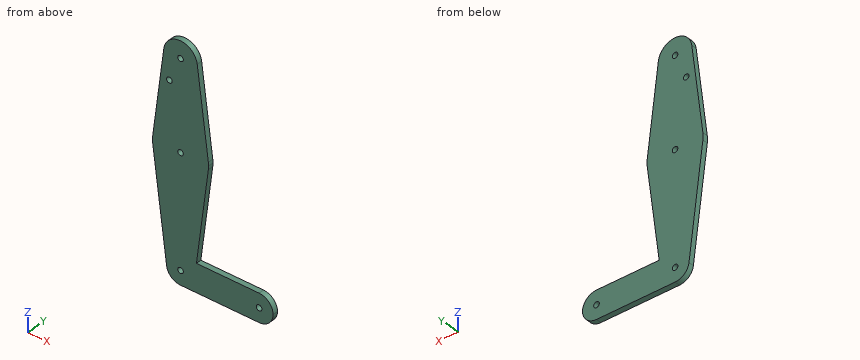
from build123d import *

# Parameters (mm, degrees)
F0_R     = 1.5875
F0_R_2   = 1.6002
F1_DEPTH = 3.048
F4_DEPTH = 3.048


# Not quite as in the source:
# - a feature of the source that left no trace in its solid (it failed there, or was rolled back) is left out


with BuildPart() as f1:
    # F0 (on Front) → F1 (new body)
    with BuildSketch(Plane.XZ):
        with BuildLine():
            ThreePointArc((-9.4502929642, 115.490625), (-0.596483242, 104.7936951058), (9.525, 114.3))
            ThreePointArc((9.525, 114.3), (9.5063048942, 114.896483242), (9.4502929642, 115.490625))
            ThreePointArc((9.4502929642, 115.490625), (0, 123.825), (-9.4502929642, 115.490625))
        make_face()
        with Locations((0, 114.3)):
            Circle(F0_R, mode=Mode.SUBTRACT)
        with BuildLine():
            ThreePointArc((9.4502929642, 115.490625), (9.5063048942, 114.896483242), (9.525, 114.3))
            ThreePointArc((9.525, 114.3), (-0.596483242, 104.7936951058), (-9.4502929642, 115.490625))
            Line((-9.4502929642, 115.490625), (-15.7504882737, 65.484375))
            ThreePointArc((-15.7504882737, 65.484375), (0, 79.375), (15.7504882737, 65.484375))
            Line((15.7504882737, 65.484375), (9.4502929642, 115.490625))
        make_face()
        with Locations((-6.3295518048, 99.7836068273)):
            Circle(F0_R, mode=Mode.SUBTRACT)
        with BuildLine():
            ThreePointArc((15.875, 63.5), (15.8438414904, 64.4941387366), (15.7504882737, 65.484375))
            ThreePointArc((15.7504882737, 65.484375), (0, 79.375), (-15.7504882737, 65.484375))
            ThreePointArc((-15.7504882737, 65.484375), (-15.875, 63.5), (-15.7504882737, 61.515625))
            ThreePointArc((-15.7504882737, 61.515625), (0, 47.625), (15.7504882737, 61.515625))
            ThreePointArc((15.7504882737, 61.515625), (15.8438414904, 62.5058612634), (15.875, 63.5))
        make_face()
        with Locations((0, 63.5)):
            Circle(F0_R, mode=Mode.SUBTRACT)
        with BuildLine():
            ThreePointArc((15.7504882737, 61.515625), (0, 47.625), (-15.7504882737, 61.515625))
            Line((-15.7504882737, 61.515625), (-7.8752441368, -0.9921875))
            ThreePointArc((-7.8752441368, -0.9921875), (-5.953125, 5.2501627579), (0, 7.9375))
            Line((0, 7.9375), (9.0002790135, 7.9375))
            Line((9.0002790135, 7.9375), (15.7504882737, 61.515625))
        make_face()
        with BuildLine():
            ThreePointArc((0, 7.9375), (-5.953125, 5.2501627579), (-7.8752441368, -0.9921875))
            ThreePointArc((-7.8752441368, -0.9921875), (-5.2501627579, -5.953125), (0, -7.9375))
            ThreePointArc((0, -7.9375), (5.2501627579, -5.953125), (7.8752441368, -0.9921875))
            ThreePointArc((7.8752441368, -0.9921875), (7.9219207452, -0.4970693683), (7.9375, 0))
            ThreePointArc((7.9375, 0), (5.6126600757, 5.6126600757), (0, 7.9375))
        make_face()
        Circle(F0_R, mode=Mode.SUBTRACT)
        with BuildLine():
            Line((7.8752441368, -0.9921875), (9.0002790135, 7.9375))
            Line((9.0002790135, 7.9375), (0, 7.9375))
            ThreePointArc((0, 7.9375), (5.6126600757, 5.6126600757), (7.9375, 0))
            ThreePointArc((7.9375, 0), (7.9219207452, -0.4970693683), (7.8752441368, -0.9921875))
        make_face()
        with BuildLine():
            Line((44.45, 7.9375), (9.0002790135, 7.9375))
            Line((9.0002790135, 7.9375), (7.8752441368, -0.9921875))
            ThreePointArc((7.8752441368, -0.9921875), (5.2501627579, -5.953125), (0, -7.9375))
            Line((0, -7.9375), (44.45, -7.9375))
            ThreePointArc((44.45, -7.9375), (36.5125, 0), (44.45, 7.9375))
        make_face()
        with BuildLine():
            ThreePointArc((52.3875, 0), (50.0626600757, 5.6126600757), (44.45, 7.9375))
            ThreePointArc((44.45, 7.9375), (36.5125, 0), (44.45, -7.9375))
            ThreePointArc((44.45, -7.9375), (50.0626600757, -5.6126600757), (52.3875, 0))
        make_face()
        with Locations((44.45, 0)):
            Circle(F0_R_2, mode=Mode.SUBTRACT)
    extrude(amount=F1_DEPTH)


with BuildPart() as f4:
    # F0 (on Front) → F4 (new body)
    with BuildSketch(Plane.XZ):
        with BuildLine():
            ThreePointArc((-9.4502929642, 115.490625), (-0.596483242, 104.7936951058), (9.525, 114.3))
            ThreePointArc((9.525, 114.3), (9.5063048942, 114.896483242), (9.4502929642, 115.490625))
            ThreePointArc((9.4502929642, 115.490625), (0, 123.825), (-9.4502929642, 115.490625))
        make_face()
        with Locations((0, 114.3)):
            Circle(F0_R, mode=Mode.SUBTRACT)
        with BuildLine():
            ThreePointArc((9.4502929642, 115.490625), (9.5063048942, 114.896483242), (9.525, 114.3))
            ThreePointArc((9.525, 114.3), (-0.596483242, 104.7936951058), (-9.4502929642, 115.490625))
            Line((-9.4502929642, 115.490625), (-15.7504882737, 65.484375))
            ThreePointArc((-15.7504882737, 65.484375), (0, 79.375), (15.7504882737, 65.484375))
            Line((15.7504882737, 65.484375), (9.4502929642, 115.490625))
        make_face()
        with Locations((-6.3295518048, 99.7836068273)):
            Circle(F0_R, mode=Mode.SUBTRACT)
        with BuildLine():
            ThreePointArc((15.875, 63.5), (15.8438414904, 64.4941387366), (15.7504882737, 65.484375))
            ThreePointArc((15.7504882737, 65.484375), (0, 79.375), (-15.7504882737, 65.484375))
            ThreePointArc((-15.7504882737, 65.484375), (-15.875, 63.5), (-15.7504882737, 61.515625))
            ThreePointArc((-15.7504882737, 61.515625), (0, 47.625), (15.7504882737, 61.515625))
            ThreePointArc((15.7504882737, 61.515625), (15.8438414904, 62.5058612634), (15.875, 63.5))
        make_face()
        with Locations((0, 63.5)):
            Circle(F0_R, mode=Mode.SUBTRACT)
        with BuildLine():
            ThreePointArc((15.7504882737, 61.515625), (0, 47.625), (-15.7504882737, 61.515625))
            Line((-15.7504882737, 61.515625), (-7.8752441368, -0.9921875))
            ThreePointArc((-7.8752441368, -0.9921875), (-5.953125, 5.2501627579), (0, 7.9375))
            Line((0, 7.9375), (9.0002790135, 7.9375))
            Line((9.0002790135, 7.9375), (15.7504882737, 61.515625))
        make_face()
        with BuildLine():
            ThreePointArc((0, 7.9375), (-5.953125, 5.2501627579), (-7.8752441368, -0.9921875))
            ThreePointArc((-7.8752441368, -0.9921875), (-5.2501627579, -5.953125), (0, -7.9375))
            ThreePointArc((0, -7.9375), (5.2501627579, -5.953125), (7.8752441368, -0.9921875))
            ThreePointArc((7.8752441368, -0.9921875), (7.9219207452, -0.4970693683), (7.9375, 0))
            ThreePointArc((7.9375, 0), (5.6126600757, 5.6126600757), (0, 7.9375))
        make_face()
        Circle(F0_R, mode=Mode.SUBTRACT)
        with BuildLine():
            Line((7.8752441368, -0.9921875), (9.0002790135, 7.9375))
            Line((9.0002790135, 7.9375), (0, 7.9375))
            ThreePointArc((0, 7.9375), (5.6126600757, 5.6126600757), (7.9375, 0))
            ThreePointArc((7.9375, 0), (7.9219207452, -0.4970693683), (7.8752441368, -0.9921875))
        make_face()
        with BuildLine():
            Line((44.45, 7.9375), (9.0002790135, 7.9375))
            Line((9.0002790135, 7.9375), (7.8752441368, -0.9921875))
            ThreePointArc((7.8752441368, -0.9921875), (5.2501627579, -5.953125), (0, -7.9375))
            Line((0, -7.9375), (44.45, -7.9375))
            ThreePointArc((44.45, -7.9375), (36.5125, 0), (44.45, 7.9375))
        make_face()
        with BuildLine():
            ThreePointArc((52.3875, 0), (50.0626600757, 5.6126600757), (44.45, 7.9375))
            ThreePointArc((44.45, 7.9375), (36.5125, 0), (44.45, -7.9375))
            ThreePointArc((44.45, -7.9375), (50.0626600757, -5.6126600757), (52.3875, 0))
        make_face()
        with Locations((44.45, 0)):
            Circle(F0_R_2, mode=Mode.SUBTRACT)
    extrude(amount=F4_DEPTH)


solid = f4.part
Work out the finished part from the listing and answer in its coordinate system (mm). Give positions to 0.01 mm unless a question says otherwise; leave off trailing zeros. Order: outer loops, then holes, each group sorted by start corner. A loop starts at its lowest first (then second) coordinate and runs counter-clockwise, first axis right, second up. Notation, with made-up numbers: (89.5, -7.5) -> (146.5, -7.5) arc R22 ccw to (146.5, 9.5) -> close; hole circle Ø4 at (5.5, 40). An arc over 180 degrees is marked (long way). One line per item, written item: value.
Item 1: Find section C-C, the plane x = 22. Give the vertices of the cut face in (y, z).
Answer sheet:
outline: (-3.05, -7.94) -> (0, -7.94) -> (0, 7.94) -> (-3.05, 7.94) -> close
Item 2: Find section B-B, the plane y = -2.1. State how many separate pieces and enclosed holes the cut face has, plus the area to 3 significant figures.
Answer sheet:
separate pieces: 1
enclosed holes: 5
area: 3,710 mm²
Item 3: Straight lines are drawn through the part: probe 1 along Z at (x, y) = (0, -1.95) (1 decimal); probe 2 along Z at (x, y) = (-0.5, -1.35); probe 3 along Z at (x, y) = (22, -2.6). For each, find the intervals that lie inside material, in ascending order.
Answer sheet:
probe 1: -7.9 to -1.6, 1.6 to 61.9, 65.1 to 112.7, 115.9 to 123.8
probe 2: -7.92 to -1.51, 1.51 to 61.99, 65.01 to 112.79, 115.81 to 123.81
probe 3: -7.94 to 7.94
Item 4: Find section D-D, the plane z = 29.5. Give the vertices of the cut face in (x, y), plus the area to 3 significant figures.
Answer sheet:
outline: (-11.72, -3.05) -> (11.72, -3.05) -> (11.72, 0) -> (-11.72, 0) -> close
area: 71.4 mm²
Item 5: Find section A-A, the plane z = 114.3. Give the vertices of the cut face in (x, y), plus the area to 3 significant figures.
Answer sheet:
outline: (-9.6, -3.05) -> (-1.59, -3.05) -> (-1.59, 0) -> (-9.6, 0) -> close; (1.59, -3.05) -> (9.6, -3.05) -> (9.6, 0) -> (1.59, 0) -> close
area: 48.8 mm²
Item 6: A flat-ended cylindrical pin translates along its axis: P1, Ø0.9, axis at x = 35, y = -1.5, coming from the +Z side. Find the tip coordinate at first contact, or state that the pin passes through.
Answer sheet:
P1: z = 7.94
